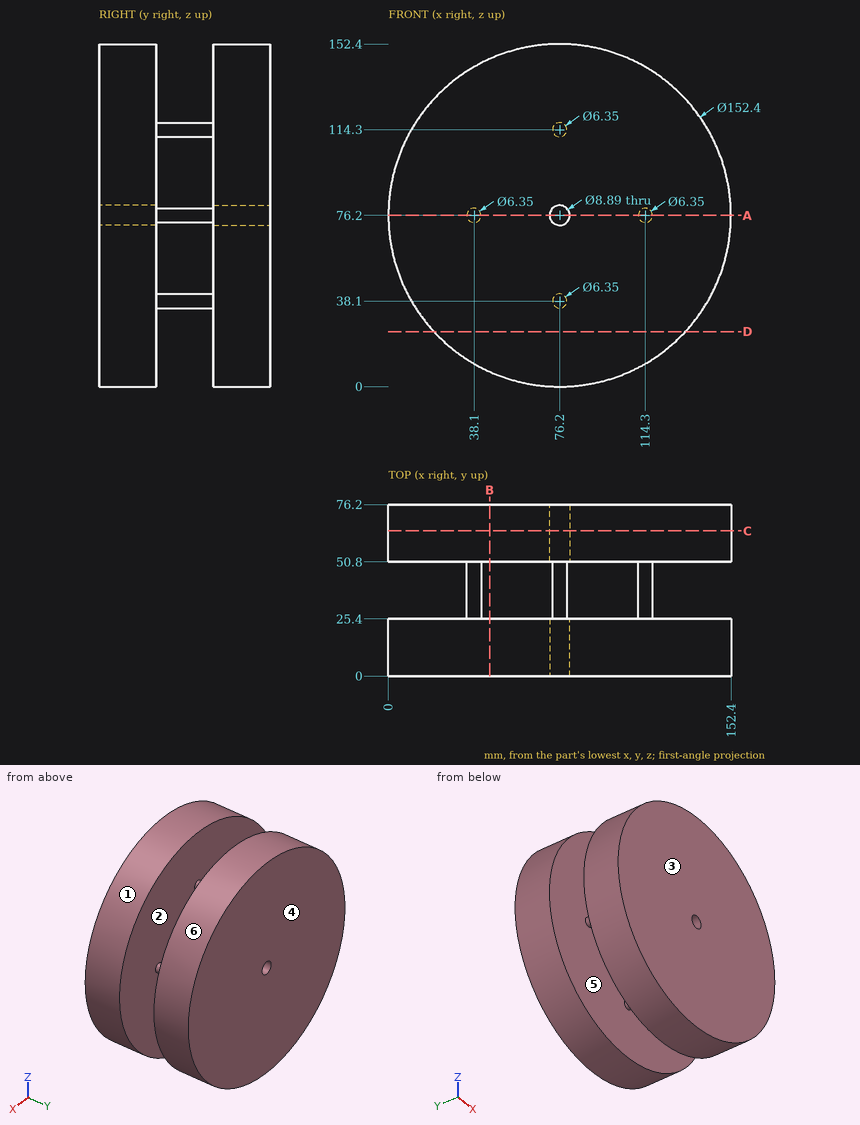
Source: three-view drawing plus pictorial views. Frame: mm from the lowest corner of the part. A direction names the side the tool comes from. Give positions to 0.01 mm unless a question says otherwise; leave off trailing zeros. Loops run counter-clockwise (first coordinate to the right, second up) from the corner with the lowest first, then second, coordinate; pieces in that order, holes last. Notation, with made-up numbers: (-35, 81) -> (15, 81) arc R17 ccw to (15, 85) -> close; hole circle Ø7 at (-39.75, 69.25). An arc over 180 degrees is marked (long way). Use a Markdown table: item, result. Add a question column.
(1) Section query C-C (y = 64.5). Output: boundary loops of the cut face in (x, z) (3 decimals).
(2) Section query B-B (x = 45). Output: boundary loops of the cut face in (y, z), then the cut area to 3 significant figures.
(3) Ray query, line 1 (Y direction, x = 56, z = 107.5); line 2 (Z direction, x = 76, y = 65). Return the intervals inside material, ascending.
(4) Section query D-D (z = 24.5). Output: boundary loops of the cut face in (x, y), then the cut area to 3 significant figures.
(5) Access query for the marked faces 5 and 6. Directions: +Z, -Z, +X, -X, +Y, -Y. A direction counts if a zero-diameter tool reaches every point of the face in a straight line with its end or side. Return the directions, or none.
(6) First-contact query: pin 1 Ø8 at (x, y) = (126, 28.5) entering from -Z; pin 2 Ø1 at (x, y) = (30.5, 9.5) entering from +Z; pin 3 Ø1.5 at (y, z) = (10, 85) entering from +X. Flat tips, straight axial feed; report the tip coordinate or a pass-through.
(7) Section query A-A (z = 76.2). Output: boundary loops of the cut face in (x, y) (3 decimals), then the cut area to 3 significant figures.
(8) Pull-direction query (Y, two-part tool) for the marked faces 1, 2, 3 and 4; classes: +Y half, -Y half, draft (parallel to the pull), parting line (faces both ways), or undercut.
Checked values:
| question | item | result |
|---|---|---|
| 1 | outline | circle Ø152.4 at (76.2, 76.2); hole circle Ø8.89 at (76.2, 76.2) |
| 2 | outline | (0, 6.68) -> (25.4, 6.68) -> (25.4, 145.72) -> (0, 145.72) -> close; (50.8, 6.68) -> (76.2, 6.68) -> (76.2, 145.72) -> (50.8, 145.72) -> close |
| 2 | area | 7,060 mm^2 |
| 3 | line 1 | 0 to 25.4, 50.8 to 76.2 |
| 3 | line 2 | 0 to 71.76, 80.64 to 152.4 |
| 4 | outline | (20.22, 0) -> (132.18, 0) -> (132.18, 25.4) -> (20.22, 25.4) -> close; (20.22, 50.8) -> (132.18, 50.8) -> (132.18, 76.2) -> (20.22, 76.2) -> close |
| 4 | area | 5,690 mm^2 |
| 5 | face 5 | none |
| 5 | face 6 | +Y, -Y |
| 6 | pin 1 | z = 16.44 |
| 6 | pin 2 | z = 137.55 |
| 6 | pin 3 | x = 151.97 |
| 7 | outline | (0, 0) -> (71.755, 0) -> (71.755, 25.4) -> (41.275, 25.4) -> (41.275, 50.8) -> (71.755, 50.8) -> (71.755, 76.2) -> (0, 76.2) -> (0, 50.8) -> (34.925, 50.8) -> (34.925, 25.4) -> (0, 25.4) -> close; (80.645, 0) -> (152.4, 0) -> (152.4, 25.4) -> (117.475, 25.4) -> (117.475, 50.8) -> (152.4, 50.8) -> (152.4, 76.2) -> (80.645, 76.2) -> (80.645, 50.8) -> (111.125, 50.8) -> (111.125, 25.4) -> (80.645, 25.4) -> close |
| 7 | area | 7,610 mm^2 |
| 8 | face 1 | draft |
| 8 | face 2 | undercut |
| 8 | face 3 | -Y half |
| 8 | face 4 | +Y half |
